from build123d import *

# Parameters (mm, degrees)
BOSS_EXTRUDE1_DEPTH = 10
SKETCH3_R           = 1.73
CUT_EXTRUDE1_DEPTH  = 10


with BuildPart() as part:
    # Sketch1 → Boss-Extrude1 (new body)
    with BuildSketch(Plane.XY):
        Polygon((-12.797368251, 238.318722846), (-32.797368251, 238.318722846), (-32.797368251, 228.318722846), (-22.797368251, 228.318722846), (-22.797368251, 155.639230922), (-22.797368251, 144.092225538), (-12.797368251, 149.86572823), align=None)
        Polygon((-32.797368251, 228.318722846), (-32.797368251, 238.318722846), (-52.797368251, 238.318722846), (-52.797368251, 149.86572823), (-42.797368251, 144.092225538), (-42.797368251, 155.639230922), (-42.797368251, 228.318722846), align=None)
        Polygon((-32.797368251, 138.318722846), (-32.797368251, 149.86572823), (-37.797368251, 152.752479576), (-42.797368251, 155.639230922), (-42.797368251, 144.092225538), align=None)
        Polygon((-27.797368251, 152.752479576), (-32.797368251, 149.86572823), (-32.797368251, 138.318722846), (-22.797368251, 144.092225538), (-22.797368251, 155.639230922), align=None)
    extrude(amount=BOSS_EXTRUDE1_DEPTH)

    # Sketch3 → Cut-Extrude1 (cut)
    with BuildSketch(Plane.XY.offset(10)):
        with Locations((-47.742368251, 228.318722846)):
            Circle(SKETCH3_R)
        with Locations((-47.742368251, 204.258722846)):
            Circle(SKETCH3_R)
        with Locations((-17.852368251, 204.258722846)):
            Circle(SKETCH3_R)
        with Locations((-17.852368251, 228.318722846)):
            Circle(SKETCH3_R)
    extrude(amount=-CUT_EXTRUDE1_DEPTH, mode=Mode.SUBTRACT)


solid = part.part
The model under review builds one solid part; all positions refer to its coordinate system, in mm. A direction names the side the tool comes from. Give positions to 0.01 mm unless a question says otherwise; leave off trailing zeros. Write each loop counter-clockwise with the first axis right and the second up, starting at its lowest first coordinate (ties: lowest second). Pieces come first, ordered by that corner, then holes. Notation, with made-up numbers: M 27.5,-12.75 L 56.5,-12.75 A10 cw 56.5,-1.75 Z; hole C -2.5,42.5 d3. An arc over 180 degrees is marked long. One line per question, with ' | ' between items. Start each with the question number.
Item 1: We need section D-D on x = -44.5. Write out the cut boundary in (y, z), plus the area to 3 significant figures.
Item 2: We need section A-A on y = 175. Write out the cut boundary in (x, z).
Item 3: For pin 1 (3 mm diameter, centred on x = -21.5, z = 6.5, fed in from -Y), flat-tipped, find the tip position at first contact; note if it passes through.
Item 4: We need section C-C on z = 3.25. Write out the cut boundary in (x, y).
Item 5: Draft analysis for pull direction X (two halves, no side actions). For faces 1 (the flat face through (-22.797, 192, 5)), 2 (the flat face through (-20, 189, 10)), 3 (the flat face through (-22.94, 144.01, 4.93)), 4 (the flat face through (-52.797, 195, 5)), state which applies: released by +X, released by -X, zero draft, split by the parting line, or undercut.
Item 6: We need section B-B on x = -30.5. Write out the cut boundary in (y, z).
Item 7: Wall thickness on line 1 (X direction, y = 210.5, z = 7.5); line 2 (Y direction, x = -49, z = 3.5); line 3 (X direction, y = 203, z = 5.75): over which ranges is each line inside the solid? List them lowest first. Write a range as from..to.
Item 8: For faces 5 (the flat face through (-33, 238.319, 5)), 6 (the flat face through (-33, 228.319, 5)), list the 3-axis set-ups (+Z, -Z, +X, -X, +Y, -Y) from which the entire face can be reached by the end or side of a thin tool; tool diameter is ignored.
Results found:
1) outline: M 145.08,0 L 238.32,0 L 238.32,10 L 145.08,10 Z | area: 932 mm2
2) outline: M -52.8,0 L -42.8,0 L -42.8,10 L -52.8,10 Z; M -22.8,0 L -12.8,0 L -12.8,10 L -22.8,10 Z
3) pin 1: stops at y = 143.98
4) outline: M -52.8,149.87 L -32.8,138.32 L -12.8,149.87 L -12.8,238.32 L -52.8,238.32 Z; hole C -47.74,204.26 d3.46; hole C -47.74,228.32 d3.46; hole M -42.8,155.64 L -32.8,149.87 L -22.8,155.64 L -22.8,228.32 L -42.8,228.32 Z; hole C -17.85,204.26 d3.46; hole C -17.85,228.32 d3.46
5) face 1: undercut | face 2: zero draft | face 3: released by +X | face 4: released by -X
6) outline: M 139.65,0 L 151.19,0 L 151.19,10 L 139.65,10 Z; M 228.32,0 L 238.32,0 L 238.32,10 L 228.32,10 Z
7) line 1: x = -52.8..-42.8, -22.8..-12.8 | line 2: y = 147.67..203.07, 205.45..227.13, 229.51..238.32 | line 3: x = -52.8..-48.93, -46.56..-42.8, -22.8..-19.04, -16.67..-12.8
8) face 5: +Z, -Z, +X, -X, +Y | face 6: +Z, -Z
